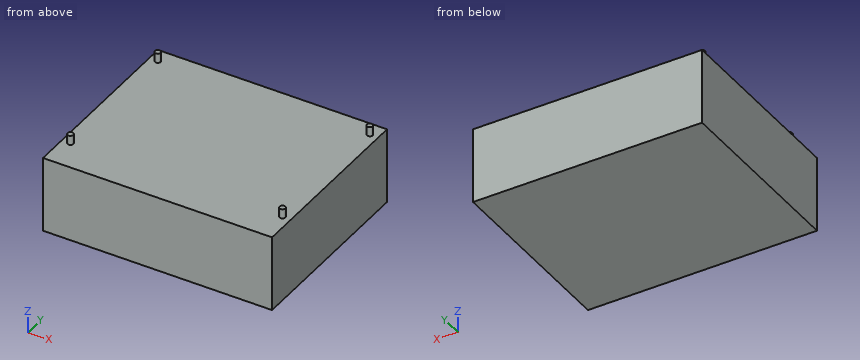
from build123d import *

# Parameters (mm, degrees)
SKETCH_1_W          = 121
SKETCH_1_H          = 100
EXTRUDE_1_DEPTH     = 40
SKETCH_2_R          = 1.5
EXTRUDE_2_DEPTH     = 5
SKETCH_3_W          = 117
SKETCH_3_H          = 96
CUT_EXTRUDE_1_DEPTH = 38
SKETCH_4_W          = 117
SKETCH_4_H          = 96
EXTRUDE_3_DEPTH     = 2


with BuildPart() as part:
    # 草图1 → 凸台-拉伸1 (new body)
    with BuildSketch(Plane.XY):
        with Locations((-60.5, 50)):
            Rectangle(SKETCH_1_W, SKETCH_1_H)
    extrude(amount=EXTRUDE_1_DEPTH)

    # 草图2 → 凸台-拉伸2 (add)
    with BuildSketch(Plane.XY.offset(40)):
        with Locations((-116.5, 92.5)):
            Circle(SKETCH_2_R)
        with Locations((-4.5, 92.5)):
            Circle(SKETCH_2_R)
        with Locations((-116.5, 16.5)):
            Circle(SKETCH_2_R)
        with Locations((-4.5, 16.5)):
            Circle(SKETCH_2_R)
    extrude(amount=EXTRUDE_2_DEPTH)

    # 草图3 → 切除-拉伸1 (cut)
    with BuildSketch(Plane(origin=(0, 0, 0), x_dir=(-1, 0, 0), z_dir=(0, 0, -1))):
        with Locations((60.5, 50)):
            Rectangle(SKETCH_3_W, SKETCH_3_H)
    extrude(amount=-CUT_EXTRUDE_1_DEPTH, mode=Mode.SUBTRACT)

    # 草图4 → 凸台-拉伸3 (add)
    with BuildSketch(Plane(origin=(0, 0, 0), x_dir=(-1, 0, 0), z_dir=(0, 0, -1))):
        with Locations((60.5, 50)):
            Rectangle(SKETCH_4_W, SKETCH_4_H)
    extrude(amount=-EXTRUDE_3_DEPTH)


solid = part.part
Here's how the part is built. I have some questions about the finished solid (model axes, mm). Coordinates: 2 decimals unless noted, no trailing zeros. Loops run counter-clockwise (first coordinate to the right, second up) from the corner with the lowest first, then second, coordinate; pieces in that order, holes last. Notation, with made-up numbers: (36.25, -8) -> (59.25, -8) arc R6 cw to (59.25, 3) -> close; hole circle Ø5 at (10, 16.5). An arc over 180 degrees is marked (long way). Use one line per item in the form item = value. Start each with the question number.
(1) Please list where these lines run through material, in increasing order: line 1 along Y through (x, z) = (-13, 2.5); line 2 along X through (y, z) = (79.5, 14); line 3 along Z through (x, y) = (-85.5, 72).
(2) Will this pin go through, and if not, where does the flat tip stop? pin 1 (4 mm diameter, centred on x = -80, y = 53, fed in from +Z).
(3) If we section it at B-B (y = 92.5): Please give me the cut outline in (x, z), then the cut area to 3 significant figures.
(4) If we section it at A-A (z = 24.5): Please give me the cut outline in (x, y), then the cut area to 3 significant figures.
(5) If we section it at D-D (x = -4.5): Please give me the cut outline in (y, z).
(6) If we section it at C-C (x = -49): Please give me the cut outline in (y, z), then the cut area to 3 significant figures.
Verdict:
q1.line_1 = 0 to 2, 98 to 100
q1.line_2 = -121 to -119, -2 to 0
q1.line_3 = 0 to 2, 38 to 40
q2.pin_1 = 40
q3.outline = (-121, 0) -> (0, 0) -> (0, 40) -> (-3, 40) -> (-3, 45) -> (-6, 45) -> (-6, 40) -> (-115, 40) -> (-115, 45) -> (-118, 45) -> (-118, 40) -> (-121, 40) -> close; hole (-119, 2) -> (-2, 2) -> (-2, 38) -> (-119, 38) -> close
q3.area = 658 mm²
q4.outline = (-121, 0) -> (0, 0) -> (0, 100) -> (-121, 100) -> close; hole (-119, 2) -> (-2, 2) -> (-2, 98) -> (-119, 98) -> close
q4.area = 868 mm²
q5.outline = (0, 0) -> (100, 0) -> (100, 40) -> (94, 40) -> (94, 45) -> (91, 45) -> (91, 40) -> (18, 40) -> (18, 45) -> (15, 45) -> (15, 40) -> (0, 40) -> close; hole (2, 2) -> (98, 2) -> (98, 38) -> (2, 38) -> close
q6.outline = (0, 0) -> (100, 0) -> (100, 40) -> (0, 40) -> close; hole (2, 2) -> (98, 2) -> (98, 38) -> (2, 38) -> close
q6.area = 544 mm²
